from build123d import *

# Parameters (mm, degrees)
F0_R     = 4.825
F1_DEPTH = 33
F3_DEPTH = 6.5
F4_R     = 0.2


with BuildPart() as f1:
    # F0 (on Top) → F1 (new body)
    with BuildSketch(Plane.XY):
        Circle(F0_R)
    extrude(amount=F1_DEPTH)

    # F2 (on Front) → F3 (join)
    with BuildSketch(Plane.XZ):
        with BuildLine():
            ThreePointArc((-1.5, 3.5), (0, 2), (1.5, 3.5))
            Line((1.5, 3.5), (1.5, 6.5))
            ThreePointArc((1.5, 6.5), (0, 8), (-1.5, 6.5))
            Line((-1.5, 6.5), (-1.5, 3.5))
        make_face()
    extrude(amount=F3_DEPTH)

    # F4
    f4_edges = [f1.edges().sort_by_distance(p)[0] for p in [
        (0, -6.5, 2),
        (1.5, -6.5, 5),
        (0, -6.5, 8),
        (-1.5, -6.5, 5),
    ]]
    fillet(f4_edges, radius=F4_R)

    # F5 (on Front) → F6 (revolve)
    with BuildSketch(Plane.XZ):
        with BuildLine():
            Line((0, 0), (-4.825, 0))
            ThreePointArc((-4.825, 0), (-2.5263919431, -1.1163524169), (0, -1.5))
            Line((0, -1.5), (0, 0))
        make_face()
    revolve(axis=Axis((0, 0, -1.4078605181), (0, 0, -1)))


solid = f1.part
The listing builds one solid part. Answer for the finished solid, in the listing's coordinates (mm). A direction names the side the tool comes from. Give positions to 0.01 mm unless a question says otherwise; leave off trailing zeros. Write each loop counter-clockwise with the first axis right and the second up, starting at its lowest first coordinate (ties: lowest second). Pieces come first, ordered by that corner, then holes. Notation, with made-up numbers: (-38.5, -12.5) - (3.5, -12.5) arc R12 ccw to (3.5, 8.5) - close; hole circle Ø1 at (77, 51.25). An arc over 180 degrees is marked (long way). Use a Markdown table: item, result.
1. Section A-A on x = 0 is taken. Write down the section's boundary in (y, z) (3 decimals), plus the area to 3 significant figures.
Values follow:
| item | result |
|---|---|
| outline | (-6.5, 2.2) arc R0.2 ccw to (-6.3, 2) - (-4.825, 2) - (-4.825, 0) arc R8.51 ccw to (4.825, 0) - (4.825, 33) - (-4.825, 33) - (-4.825, 8) - (-6.3, 8) arc R0.2 ccw to (-6.5, 7.8) - close |
| area | 338 mm² |
2. A tool of negligible diameter and unlimited length cuts with its end or side. For faces 1 (the flat face through (-1.5, -5, 5)), 2 (the flat face through (0, -6.5, 5)), 3 (the flat face through (1.5, -5, 5)), 4 (the cylindrical face through (0, -5, 2)), 5 (the cylindrical face through (0, -5, 8)), from which of +Z, -Z, +X, -X, +Y, -Y can it reach the whole face along a straight path? Write none if from no direction.
Values follow:
| item | result |
|---|---|
| face 1 | +Z, -Z, -X, -Y |
| face 2 | +Z, -Z, +X, -X, -Y |
| face 3 | +Z, -Z, +X, -Y |
| face 4 | -Z, -Y |
| face 5 | +Z, -Y |
3. Section D-D on z = 1 is taken. Write down the section's boundary in (x, y) (3 decimals).
Values follow:
| item | result |
|---|---|
| outline | circle Ø9.65 at (0, 0) |
4. Section C-C on y = 4 is taken. Write down the section's boundary in (x, z), plus the area to 3 significant figures.
Values follow:
| item | result |
|---|---|
| outline | (-2.7, 0) arc R7.51 ccw to (2.7, 0) - (2.7, 33) - (-2.7, 33) - close |
| area | 180 mm² |
5. Section B-B on z = 5 is taken. Write down the section's boundary in (x, y) (3 decimals).
Values follow:
| item | result |
|---|---|
| outline | (-1.5, -6.3) arc R0.2 ccw to (-1.3, -6.5) - (1.3, -6.5) arc R0.2 ccw to (1.5, -6.3) - (1.5, -4.586) arc R4.825 ccw (long way) to (-1.5, -4.586) - close |
6. Each of these flat-tipped pins is pushed along its axis until it touches: P1, Ø1.5, axis at y = 3.5, z = 7, coming from the -X side; P2, Ø4, axis at x = -3, z = 12.5, coming from the +Y side; P3, Ø5, axis at y = 3, z = 11.5, coming from the -X side. Where does it stop, or does it pass through?
Values follow:
| item | result |
|---|---|
| P1 | stops at x = -3.96 |
| P2 | stops at y = 4.72 |
| P3 | stops at x = -4.8 |
7. Find the intervals of material crossed by probe 1 along Y at (x, z) = (3.25, 11); probe 2 along Z at (x, y) = (-0.5, 0); probe 3 along Y at (x, z) = (-2, 11), in increasing order. Write a range as from..to.
Values follow:
| item | result |
|---|---|
| probe 1 | y = -3.57..3.57 |
| probe 2 | z = -1.49..33 |
| probe 3 | y = -4.39..4.39 |
